Autodesk Inventor part; units mm, degrees
ref_plane "YZ Plane" through (0, 0, 0) normal (1, 0, 0) x (0, 1, 0)
ref_plane "XZ Plane" through (0, 0, 0) normal (0, 1, 0) x (-1, 0, 0)
ref_plane "XY Plane" through (0, 0, 0) normal (0, 0, 1) x (1, 0, 0)
sketch "Sketch1" plane through (0, 0, 0) normal (0, 1, 0) x (-1, 0, 0)
  circle A0 centre (0, 0) radius 1.5875
  dimension "d0" = 3.175
extrude "Extrusion1" add sketch "Sketch1" along normal blind 19.05
thread "Thread1"
chamfer "Chamfer1" distance 0.254 angle 45 1 edges at (1.5875, 0, 0)
sketch "Sketch3" plane through (0, 0, 0) normal (1, 0, 0) x (0, 1, 0)
  point P0 (0, 0)
sketch "Sketch4" plane through (0, 19.05, 0) normal (0, 1, 0) x (1, 0, 0)
  circle A0 centre (0, 0) radius 0.9525
  dimension "d11" = 1.905
extrude "Extrusion3" add sketch "Sketch4" along normal blind 6.35
properties part number "burner_rod_1or3"
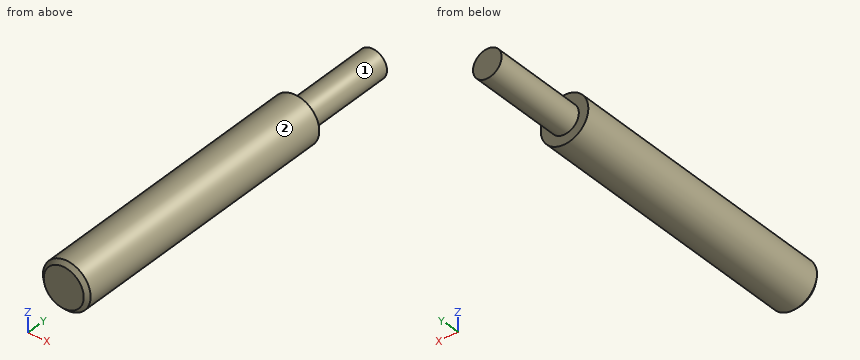
Design review of the part built by this model. Coordinates are the model's own, in mm. Face numbers are marked on the shaded views. A direction names the side the tool comes from. Give positions to 0.01 mm unless a question says otherwise; leave off trailing zeros. Order: outer loops, then holes, each group sorted by start corner. A loop starts at its lowest first (then second) coordinate and runs counter-clockwise, first axis right, second up. Notation, with made-up numbers: (33, -4.75) -> (64, -4.75) arc R25 ccw to (64, 27.25) -> close; hole circle Ø3 at (-3, 20). An arc over 180 degrees is marked (long way). Write each question's results on one line, items separated by ' | '. Start each with the question number.
Q1. For pin 1 (1.5 mm diameter, centred on x = -0.5, z = -1, fed in from -Y), flat-tipped, find the tip position at first contact; note if it passes through.
Q2. Wall thickness on L1, parallel to Y at x = 0.4, z = -0.95; L2, parallel to Z at x = 1.45, y = 7.25; L3, parallel to Z at x = -0.45, y = 11.75: over which ranges is each line inside the solid? List them lowest first. Write a range as from..to.
Q3. Add section D-D on y = 23.75. Give the boundary of the cut face in (x, z) (1 decimal), and give its area (3 significant figures).
Q4. Add section C-C on y = 16.5. Give the boundary of the cut face in (x, z) (1 decimal), and give its area (3 significant figures).
Q5. Add section A-A on x = 0. Give the boundary of the cut face in (y, z).
Q6. Machinability: for the marked faces 1 and 2, which of the approach directions +Z, -Z, +X, -X, +Y, -Y give a long, thin tool a straight path to every point of the face, cutting with its end or side? Answer none if there is none.
Q7. Add section B-B on z = 0. Give the boundary of the cut face in (x, y), and give its area (3 significant figures).
Found:
1) pin 1: stops at y = 0
2) L1: y = 0..19.05 | L2: z = -0.65..0.65 | L3: z = -1.52..1.52
3) outline: circle Ø1.9 at (0, 0) | area: 2.85 mm2
4) outline: circle Ø3.2 at (0, 0) | area: 7.92 mm2
5) outline: (0, -1.33) -> (0.25, -1.59) -> (19.05, -1.59) -> (19.05, -0.95) -> (25.4, -0.95) -> (25.4, 0.95) -> (19.05, 0.95) -> (19.05, 1.59) -> (0.25, 1.59) -> (0, 1.33) -> close
6) face 1: +Y | face 2: +Y, -Y
7) outline: (-1.59, 0.25) -> (-1.33, 0) -> (1.33, 0) -> (1.59, 0.25) -> (1.59, 19.05) -> (0.95, 19.05) -> (0.95, 25.4) -> (-0.95, 25.4) -> (-0.95, 19.05) -> (-1.59, 19.05) -> close | area: 72.5 mm2
